Here's the drawing with two shaded views (mm, measured from the low corner). I have some questions. A direction names the side the tool comes from. Round coordinates to 2 decimals unless told otherwise and drop trailing zeros. Loops run counter-clockwise (first coordinate to the right, second up) from the corner with the lowest first, then second, coordinate; pieces in that order, holes last. Notation, with made-up numbers: (86.25, 78.25) -> (98.25, 78.25) arc R29 ccw to (98.25, 103.25) -> close; hole circle Ø4 at (77.25, 64). An arc over 180 degrees is marked (long way). Use a Markdown table: item, result.
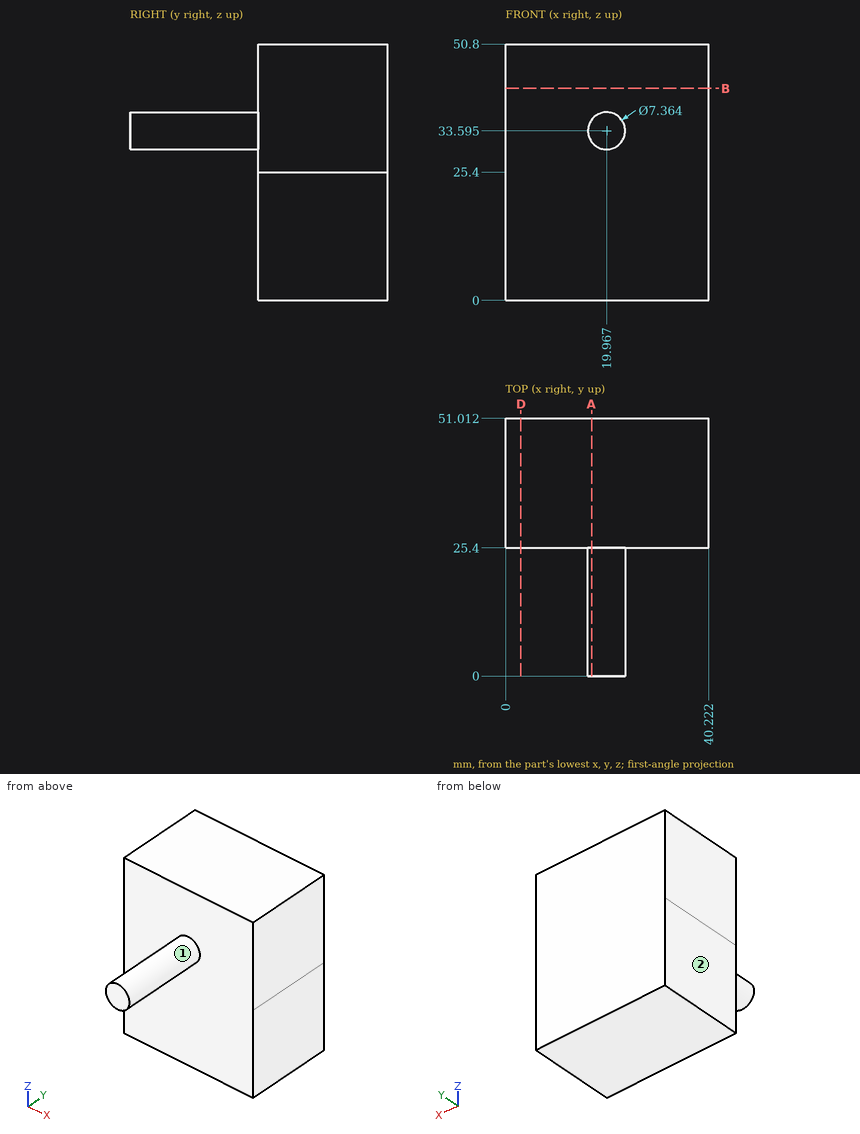
1. I want a section at B-B (z = 42). Please give me the cut outline in (x, y), plus the area to 3 significant figures.
Answer sheet:
| item | result |
|---|---|
| outline | (0, 25.4) -> (40.22, 25.4) -> (40.22, 51.01) -> (0, 51.01) -> close |
| area | 1,030 mm² |
2. Will this pin go through, and if not, where does the flat tip stop? pin 1 Ø20 at (x, z) = (20, 17) entering from -Y.
Answer sheet:
| item | result |
|---|---|
| pin 1 | stops at y = 25.4 |
3. I want a section at D-D (x = 3). Please give me the cut outline in (y, z).
Answer sheet:
| item | result |
|---|---|
| outline | (25.4, 0) -> (51.01, 0) -> (51.01, 50.8) -> (25.4, 50.8) -> close |
4. Which directions (+Z, -Z, +X, -X, +Y, -Y) give clear straight access to the entire face, cutting with the end or side of a thin tool? Please do the marked faces 1 and 2.
Answer sheet:
| item | result |
|---|---|
| face 1 | -Y |
| face 2 | +Z, -Z, -X, +Y, -Y |
5. I want a section at A-A (x = 17). Please give me the cut outline in (y, z) (1 decimal).
Answer sheet:
| item | result |
|---|---|
| outline | (0, 31.4) -> (25.4, 31.4) -> (25.4, 0) -> (51, 0) -> (51, 50.8) -> (25.4, 50.8) -> (25.4, 35.8) -> (0, 35.8) -> close |
6. I need wall thicknesses on line 1 (Y direction, x = 37, z = 9). Which ranges of the line are inside material? Lowest first, please.
Answer sheet:
| item | result |
|---|---|
| line 1 | y = 25.4 to 51.01 |
